from build123d import *

# Parameters (mm, degrees)
SKETCH1_W           = 628.65
SKETCH1_H           = 165.1
BOSS_EXTRUDE1_DEPTH = 12.7
CUT_EXTRUDE1_DEPTH  = 12.7
FILLET1_R           = 6.35


with BuildPart() as part:
    # Sketch1 → Boss-Extrude1 (new body)
    with BuildSketch(Plane(origin=(0, 0, 0), x_dir=(1, 0, 0), z_dir=(0, 1, 0))):
        Rectangle(SKETCH1_W, SKETCH1_H)
    extrude(amount=BOSS_EXTRUDE1_DEPTH)

    # Sketch2 → Cut-Extrude1 (cut)
    with BuildSketch(Plane.XZ):
        Polygon((149.225, 82.55), (250.825, 82.55), (244.475, 60.96), (155.575, 60.96), align=None)
    extrude(amount=-CUT_EXTRUDE1_DEPTH, mode=Mode.SUBTRACT)

    # Fillet1
    fillet1_edges = [part.edges().sort_by_distance(p)[0] for p in [
        (155.575, 6.35, 60.96),
        (149.225, 6.35, 82.55),
        (250.825, 6.35, 82.55),
        (244.475, 6.35, 60.96),
    ]]
    fillet(fillet1_edges, radius=FILLET1_R)


solid = part.part
Geometry check sheet. Reference: the model listing, model coordinates, mm. A direction names the side the tool comes from. Round coordinates to 2 decimals unless told otherwise and drop trailing zeros. Order: outer loops, then holes, each group sorted by start corner. A loop starts at its lowest first (then second) coordinate and runs counter-clockwise, first axis right, second up. Notation, with made-up numbers: M 28,29 L 80,29 A9 cw 80,46 Z; hole C 6.5,32 d11. An arc over 180 degrees is marked long. Answer in a Markdown table with one row per item. Add a question column.
Item 1: Draft check along X on faces 1 (the face through (-314.325, 6, 1)), 2 (the face through (-88, 6, 82.55)), 3 (the face through (152.426, 6.261, 71.668)). Enter one of: released by +X, released by -X, zero draft, split by the parting line, or undercut.
Item 2: Sectioned sample at A-A, the plane y = 9. Enter the section's corners in (x, z) (3 decimals), plus the area to 3 significant figures.
Item 3: Material ranges on L1, parallel to Z at x = 199, y = 2.5; L2, parallel to X at y = 3.75, z = 73.5 (3 decimals); L3, parallel to Z at x = 244, y = 11.25, recorded low to high. Write a range as [from, to].
Item 4: Set-up check for faces 4 (the face through (201, 6, 60.96)), 5 (the face through (314.325, 6, 1)): record each of +Z, -Z, +X, -X, +Y, -Y from which the full face is reachable in a straight line by a thin tool's end or side.
Item 5: Sectioned sample at B-B, the plane x = 210.5. Enter the section's corners in (y, z).
Item 6: Depth check by flat-ended pin: pin 1 Ø6 at (x, y) = (197.5, 4.5) entering from +Z. Enter the tip coordinate at first touch or a pass-through.
Filled in:
| question | item | result |
|---|---|---|
| 1 | face 1 | released by -X |
| 1 | face 2 | zero draft |
| 1 | face 3 | undercut |
| 2 | outline | M -314.325,-82.55 L 314.325,-82.55 L 314.325,82.55 L 255.576,82.55 A6.35 ccw 249.484,77.992 L 245.816,65.518 A6.35 cw 239.724,60.96 L 160.326,60.96 A6.35 cw 154.234,65.518 L 150.566,77.992 A6.35 ccw 144.474,82.55 L -314.325,82.55 Z |
| 2 | area | 102,000 mm² |
| 3 | L1 | z = [-82.55, 60.96] |
| 3 | L2 | x = [-314.325, 151.887], [248.163, 314.325] |
| 3 | L3 | z = [-82.55, 62.62] |
| 4 | face 4 | +Z, +Y, -Y |
| 4 | face 5 | +Z, -Z, +X, +Y, -Y |
| 5 | outline | M 0,-82.55 L 12.7,-82.55 L 12.7,60.96 L 0,60.96 Z |
| 6 | pin 1 | stops at z = 60.96 |
